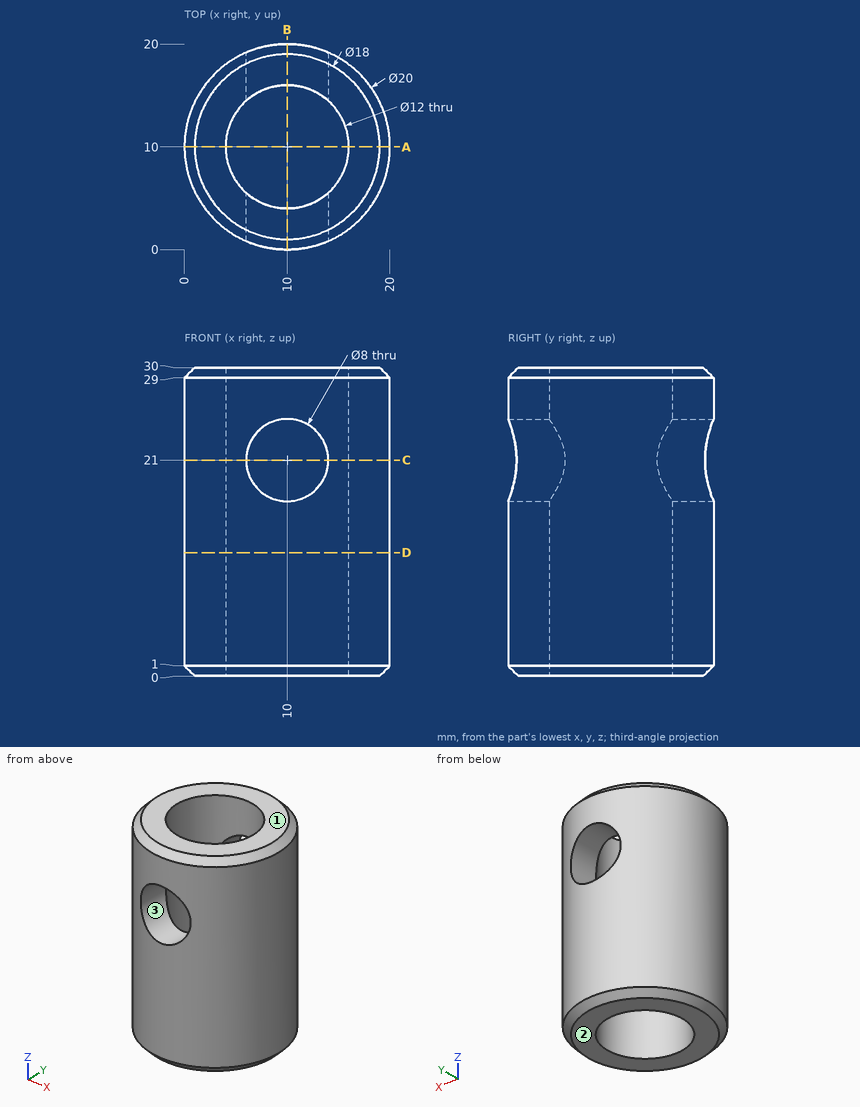
Geometry: see drawing. Coordinates: mm, zero at the bounding-box minimum. Coordinates: 2 decimals unless noted, no trailing zeros. Write each loop counter-clockwise with the first axis right and the second up, starting at its lowest first coordinate (ties: lowest second). Pieces come first, ordered by that corner, then holes.
1) Section A-A on y = 10. Output: boundary loops of the cut face in (x, z), and give its area (3 significant figures).
2) Section D-D on z = 12. Output: boundary loops of the cut face in (x, y), and give its area (3 significant figures).
3) Pin query (flat end, axial travel): pin 1 Ø10 at (y, z) = (3.5, 9) entering from +X; pin 2 Ø1.5 at (y, z) = (17, 16) entering from +X; pin 3 Ø3 at (y, z) = (17.5, 8) entering from +X. Return the tip coordinate at first contact, or that it passes through.
4) Section C-C on z = 21. Output: boundary loops of the cut face in (x, y), and give its area (3 significant figures).
5) Section B-B on x = 10. Output: boundary loops of the cut face in (y, z).
6) Material intervals for line 1 along Y through (x, z) = (9.75, 16); line 2 along Z through (x, y) = (10, 16.85); line 3 along Y through (x, z) = (6.25, 26), sorted ascending.
7) Mould query, pull axis Z, two halves, no side actions, for the marked faces 1, 2 and 3. Classes: pulls with the +Z half, pulls with the -Z half, needs draft (parallel to the pull), parting line crosses it, or undercut.
Check result:
1. outline: (0, 1) - (1, 0) - (4, 0) - (4, 30) - (1, 30) - (0, 29) - close; (16, 0) - (19, 0) - (20, 1) - (20, 29) - (19, 30) - (16, 30) - close
1. area: 238 mm2
2. outline: circle Ø20 at (10, 10); hole circle Ø12 at (10, 10)
2. area: 201 mm2
3. pin 1: stops at x = 19.89
3. pin 2: stops at x = 17.81
3. pin 3: stops at x = 18
4. outline: (6, 0.83) - (6, 5.53) arc R6 cw to (6, 14.47) - (6, 19.17) arc R10 ccw to start; (14, 0.83) arc R10 ccw to (14, 19.17) - (14, 14.47) arc R6 cw to (14, 5.53) - close
4. area: 134 mm2
5. outline: (0, 1) - (1, 0) - (4, 0) - (4, 17) - (0, 17) - close; (0, 25) - (4, 25) - (4, 30) - (1, 30) - (0, 29) - close; (16, 0) - (19, 0) - (20, 1) - (20, 17) - (16, 17) - close; (16, 25) - (20, 25) - (20, 29) - (19, 30) - (16, 30) - close
6. line 1: y = 0 to 4.01, 15.99 to 20
6. line 2: z = 0 to 17, 25 to 30
6. line 3: y = 0.73 to 5.32, 14.68 to 19.27
7. face 1: pulls with the +Z half
7. face 2: pulls with the -Z half
7. face 3: undercut
